Build history of the part. All positions in model axes, mm. Round coordinates to 2 decimals unless told otherwise and drop trailing zeros. Loops run counter-clockwise (first coordinate to the right, second up) from the corner with the lowest first, then second, coordinate; pieces in that order, holes last. Notation, with made-up numbers: M -2.5,58 L 31.5,58 A10 cw 31.5,73 Z; hole C -39.75,-40 d2. An arc over 180 degrees is marked long. One line per item, written item: value.
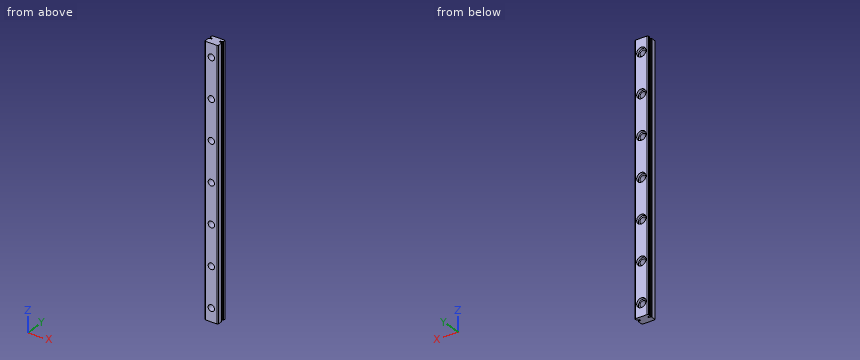
Autodesk Inventor part; units mm, degrees
ref_plane "rail_to_adjusting_block_XY" through (0, 0, -45) normal (0, 1, 0) x (1, 0, 0)
ref_plane "rail_to_adjusting_block_YZ" through (0, 0, -45) normal (1, 0, 0) x (0, 0, -1)
ref_plane "rail_to_adjusting_block_ZX" through (0, 0, -45) normal (0, 0, -1) x (0, 1, 0)
sketch "Sketch_12" plane through (0, 0, 0) normal (0, 0, 1) x (1, 0, 0)
  line L0 (-2.5, 3.7) -> (-2.5, 3.1084)
  line L1 (-2.5, 3.1084) -> (-2.3242, 3.0098)
  arc A0 (-2.1007, 2.75) -> (-2.3242, 3.0098) centre (-2.5686, 2.5736) ccw
  line L2 (-2.1007, 2.75) -> (-1.5, 2.75)
  line L3 (-1.5, 2.75) -> (-1.5, 2.25)
  line L4 (-1.5, 2.25) -> (-2.1007, 2.25)
  arc A1 (-2.3242, 1.9902) -> (-2.1007, 2.25) centre (-2.5686, 2.4264) ccw
  line L5 (-2.3242, 1.9902) -> (-2.5, 1.8917)
  line L6 (-2.5, 1.8917) -> (-2.5, 0.3)
  line L7 (-2.5, 0.3) -> (-2.2, 0)
  line L8 (-2.2, 0) -> (2.2, 0)
  line L9 (2.2, 0) -> (2.5, 0.3)
  line L10 (2.5, 0.3) -> (2.5, 1.8917)
  line L11 (2.5, 1.8917) -> (2.3242, 1.9902)
  arc A2 (2.1007, 2.25) -> (2.3242, 1.9902) centre (2.5686, 2.4263) ccw
  line L12 (2.1007, 2.25) -> (1.5, 2.25)
  line L13 (1.5, 2.25) -> (1.5, 2.75)
  line L14 (1.5, 2.75) -> (2.1007, 2.75)
  arc A3 (2.3242, 3.0098) -> (2.1007, 2.75) centre (2.5686, 2.5737) ccw
  line L15 (2.3242, 3.0098) -> (2.5, 3.1084)
  line L16 (2.5, 3.1084) -> (2.5, 3.7)
  line L17 (2.5, 3.7) -> (2.2, 4)
  line L18 (2.2, 4) -> (-2.2, 4)
  line L19 (-2.2, 4) -> (-2.5, 3.7)
extrude "Extrusion1" add sketch "Sketch_12" along normal mid plane 100
sketch "Sketch2" plane through (-2.2, 4, 50) normal (0, 1, 0) x (1, 0, 0)
  point P0 (2.2, 95)
hole "Hole1" at (0, 4, -45) direction (0, -1, 0) diameter 2.4 depth 4 counterbore diameter 3.5 counterbore depth 1
pattern_linear "Rectangular Pattern1" count 7 spacing 15 along (0, 0, 1) of "Hole1"
ref_plane "rail_to_adjusting_block_XY" through (0, 0, -45) normal (0, 1, 0) x (1, 0, 0)
ref_plane "rail_to_adjusting_block_YZ" through (0, 0, -45) normal (1, 0, 0) x (0, 0, -1)
ref_plane "rail_to_adjusting_block_ZX" through (0, 0, -45) normal (0, 0, -1) x (0, 1, 0)
ref_plane "screw_1_XY" through (0, 3, 45) normal (0, -1, 0) x (1, 0, 0)
ref_plane "screw_1_YZ" through (0, 3, 45) normal (1, 0, 0) x (0, 0, 1)
ref_plane "screw_1_ZX" through (0, 3, 45) normal (0, 0, 1) x (0, -1, 0)
ref_plane "screw_2_XY" through (0, 3, 30) normal (0, -1, 0) x (1, 0, 0)
ref_plane "screw_2_YZ" through (0, 3, 30) normal (1, 0, 0) x (0, 0, 1)
ref_plane "screw_2_ZX" through (0, 3, 30) normal (0, 0, 1) x (0, -1, 0)
ref_plane "screw_3_XY" through (0, 3, 15) normal (0, -1, 0) x (1, 0, 0)
ref_plane "screw_3_YZ" through (0, 3, 15) normal (1, 0, 0) x (0, 0, 1)
ref_plane "screw_3_ZX" through (0, 3, 15) normal (0, 0, 1) x (0, -1, 0)
ref_plane "screw_4_XY" through (0, 3, 0) normal (0, -1, 0) x (1, 0, 0)
ref_plane "screw_4_YZ" through (0, 3, 0) normal (1, 0, 0) x (0, 0, 1)
ref_plane "screw_4_ZX" through (0, 3, 0) normal (0, 0, 1) x (0, -1, 0)
ref_plane "screw_5_XY" through (0, 3, -15) normal (0, -1, 0) x (1, 0, 0)
ref_plane "screw_5_YZ" through (0, 3, -15) normal (1, 0, 0) x (0, 0, 1)
ref_plane "screw_5_ZX" through (0, 3, -15) normal (0, 0, 1) x (0, -1, 0)
ref_plane "screw_6_XY" through (0, 3, -30) normal (0, -1, 0) x (1, 0, 0)
ref_plane "screw_6_YZ" through (0, 3, -30) normal (1, 0, 0) x (0, 0, 1)
ref_plane "screw_6_ZX" through (0, 3, -30) normal (0, 0, 1) x (0, -1, 0)
ref_plane "screw_7_XY" through (0, 3, -45) normal (0, -1, 0) x (1, 0, 0)
ref_plane "screw_7_YZ" through (0, 3, -45) normal (1, 0, 0) x (0, 0, 1)
ref_plane "screw_7_ZX" through (0, 3, -45) normal (0, 0, 1) x (0, -1, 0)
ref_plane "to_block_XY" through (0, 4, 25) normal (0, 0, 1) x (1, 0, 0)
ref_plane "to_block_YZ" through (0, 4, 25) normal (1, 0, 0) x (0, 1, 0)
ref_plane "to_block_ZX" through (0, 4, 25) normal (0, 1, 0) x (0, 0, 1)
ref_plane "to_block_2_XY" through (0, 4, -25) normal (0, 0, 1) x (1, 0, 0)
ref_plane "to_block_2_YZ" through (0, 4, -25) normal (1, 0, 0) x (0, 1, 0)
ref_plane "to_block_2_ZX" through (0, 4, -25) normal (0, 1, 0) x (0, 0, 1)
ref_plane "to_kue_XY" through (0, 0, 0) normal (0, 1, 0) x (1, 0, 0)
ref_plane "to_kue_YZ" through (0, 0, 0) normal (1, 0, 0) x (0, 0, -1)
ref_plane "to_kue_ZX" through (0, 0, 0) normal (0, 0, -1) x (0, 1, 0)
properties part number "SSE2B6-100_r"
Item 1: Wall check: line 1 along X through (y, z) = (1.55, -15); line 2 along X through (y, z) = (3.55, 30); line 3 along X through (y, z) = (2.4, 19). Give the ranges that are in metal, low to high.
Check values:
line 1: x = -2.5 to -1.2, 1.2 to 2.5
line 2: x = -2.5 to -1.75, 1.75 to 2.5
line 3: x = -1.5 to 1.5
Item 2: Slice it at B-B, the plane y = 0.9. Give the cut face in (x, z).
Check values:
outline: M -2.5,-50 L 2.5,-50 L 2.5,50 L -2.5,50 Z; hole C 0,-45 d2.4; hole C 0,-30 d2.4; hole C 0,-15 d2.4; hole C 0,0 d2.4; hole C 0,15 d2.4; hole C 0,30 d2.4; hole C 0,45 d2.4
Item 3: Slice it at C-C, the plane x = 0. Give the number of separate pieces and of enclosed holes in the cut face, and give its area (3 significant figures).
Check values:
separate pieces: 8
enclosed holes: 0
area: 325 mm2
Item 4: Drop a flat-ended pin along its axis: P1, Ø3, axis at x = 0, z = 30, coming from the +Y side. Give the stop position or say it passes through.
Check values:
P1: stops at y = 3
